The model under review builds one solid part; all positions refer to its coordinate system, in mm. A direction names the side the tool comes from. Coordinates: 2 decimals unless noted, no trailing zeros. Loops run counter-clockwise (first coordinate to the right, second up) from the corner with the lowest first, then second, coordinate; pieces in that order, holes last. Notation, with made-up numbers: M -36.5,-7.75 L -30.5,-7.75 A21 cw -30.5,-2.75 Z; hole C -8.5,-25.75 d10. An arc over 180 degrees is marked long. Return JSON: item names as keys, results as strings.
```python
from build123d import *

# Parameters (mm, degrees)
F2_R          = 2.38125
F3_DEPTH      = 45.594
F4_R          = 21.082
F5_DEPTH      = 21.083
F5_DEPTH_BACK = 21.083


with BuildPart() as f1:
    # F0 (on Front) → F1 (revolve)
    with BuildSketch(Plane.XZ):
        Polygon((-17.272, 0), (0, 0), (0, 45.593), (-21.082, 45.593), (-21.082, 22.352), (-17.272, 22.352), align=None)
    revolve(axis=Axis((0, 0, 22.7965), (0, 0, -1)))

    # F2 (on face) → F3 (cut, through all)
    with BuildSketch(Plane(origin=(0, 0, 0), x_dir=(1, 0, 0), z_dir=(0, 0, -1))):
        Circle(F2_R)
    extrude(amount=-F3_DEPTH, mode=Mode.SUBTRACT)

    # F4 (on Front) → F5 (cut, two sides)
    with BuildSketch(Plane.XZ) as f5_sk:
        with Locations((0, 50.7746)):
            Circle(F4_R)
    extrude(amount=-F5_DEPTH, mode=Mode.SUBTRACT)
    extrude(f5_sk.sketch, amount=F5_DEPTH_BACK, mode=Mode.SUBTRACT)


solid = f1.part
```
1. Machinability: for faces 4 (the face through (-1.89, 1.45, 14.7)), 5 (the face through (2.248, 17.125, 11.02)), which of the approach directions +Z, -Z, +X, -X, +Y, -Y give a long, thin tool a straight path to every point of the face, cutting with its end or side? Answer none if there is none.
Check values:
{"face 4": "+Z, -Z", "face 5": "-Z"}
2. Add section A-A on x = 0. Give the boundary of the cut face in (y, z).
Check values:
{"outline": "M -21.08,22.35 L -17.27,22.35 L -17.27,0 L -2.38,0 L -2.38,29.69 L -21.08,29.69 Z; M 2.38,0 L 17.27,0 L 17.27,22.35 L 21.08,22.35 L 21.08,29.69 L 2.38,29.69 Z"}
3. The part is to be moulded in two halves that separate along X. For faces 1 (the face through (-20.11, 6.33, 31.23)), 2 (the face through (-0.39, -4.98, 29.696)), 3 (the face through (0, -4, 0)), say which applies: released by +X, released by -X, zero draft, split by the parting line, or undercut.
Check values:
{"face 1": "split by the parting line", "face 2": "undercut", "face 3": "zero draft"}
4. To check wall thickness, follow line 1 (Y direction, x = 0, z = 17.5); line 2 (Z direction, x = -2.5, y = 0); line 3 (X direction, y = 2, z = 13). State the ranges of each line that lie inside material, in increasing order.
Check values:
{"line 1": "-17.27 to -2.38, 2.38 to 17.27", "line 2": "0 to 29.84", "line 3": "-17.16 to -1.29, 1.29 to 17.16"}
5. Add section D-D on y = -13. Give the boundary of the cut face in (x, z), plus the area to 3 significant figures.
Check values:
{"outline": "M -16.6,22.35 L -11.37,22.35 L -11.37,0 L 11.37,0 L 11.37,22.35 L 16.6,22.35 L 16.6,37.77 A21.08 cw -16.6,37.77 Z", "area": "833 mm²"}
6. Insertion check: pin 1 Ø2 at (x, z) = (-7.5, 8.5) entering from -Y; pin 2 Ø10 at (x, y) = (9, -13.5) entering from +Z; pin 3 Ø5 at (y, z) = (-5, 7) entering from +X. Each pin has a flat end and moves straight along its axis. Give the tip position at first contact, or say it passes through.
Check values:
{"pin 1": "y = -16", "pin 2": "z = 35.01", "pin 3": "x = 17.09"}
7. Add section C-C on z = 19. Give the boundary of the cut face in (x, y).
Check values:
{"outline": "C 0,0 d34.54; hole C 0,0 d4.76"}
8. Add section B-B on y = 0. Give the boundary of the cut face in (x, z), plus the area to 3 significant figures.
Check values:
{"outline": "M -21.08,22.35 L -17.27,22.35 L -17.27,0 L -2.38,0 L -2.38,29.83 A21.08 cw -20.44,45.59 L -21.08,45.59 Z; M 2.38,0 L 17.27,0 L 17.27,22.35 L 21.08,22.35 L 21.08,45.59 L 20.44,45.59 A21.08 cw 2.38,29.83 Z", "area": "1,130 mm²"}
